Autodesk Inventor part; units mm, degrees
ref_plane "YZ Plane" through (0, 0, 0) normal (1, 0, 0) x (0, 1, 0)
ref_plane "XZ Plane" through (0, 0, 0) normal (0, 1, 0) x (-1, 0, 0)
ref_plane "XY Plane" through (0, 0, 0) normal (0, 0, 1) x (1, 0, 0)
sketch "Sketch1" plane through (0, 0, 0) normal (0, 0, 1) x (1, 0, 0)
  line L0 (25.4, -76.2) -> (25.4, 76.2)
  line L1 (25.4, 76.2) -> (-25.4, 76.2)
  line L2 (-25.4, 76.2) -> (-25.4, -76.2)
  line L3 (-25.4, -76.2) -> (25.4, 76.2) construction
  line L4 (25.4, -76.2) -> (-25.4, 76.2) construction
  line L5 (29.3687, -76.2) -> (29.3687, 80.1688)
  line L6 (29.3687, 80.1688) -> (-29.3687, 80.1688)
  line L7 (-29.3687, 80.1688) -> (-29.3687, -76.2)
  line L8 (-29.3687, -80.1688) -> (29.3687, 80.1688) construction
  line L9 (29.3687, -80.1688) -> (-29.3687, 80.1688) construction
  line L10 (-25.4, -76.2) -> (-29.3687, -76.2)
  line L11 (25.4, -76.2) -> (29.3687, -76.2)
  point P0 (0, 0)
  dimension "d2" = 3.9688
  dimension "d3" = 3.9688
  dimension "d5" = 50.8
  dimension "d6" = 152.4
extrude "Extrusion1" add sketch "Sketch1" along normal blind 31.75
sketch "Sketch2" plane through (0, 0, 0) normal (0, 0, -1) x (-1, 0, 0)
  line L0 (-29.3687, -76.2) -> (-29.3687, 80.1688)
  line L1 (29.3687, 80.1688) -> (29.3687, -76.2)
  line L2 (-29.3687, 80.1688) -> (29.3687, 80.1688)
  line L3 (29.3687, 80.1688) -> (29.3687, -76.2)
  line L4 (29.3687, -76.2) -> (-29.3687, -76.2)
  line L5 (-29.3687, -76.2) -> (-29.3687, 80.1688)
  point P0 (0, 0)
extrude "Extrusion2" add sketch "Sketch2" along normal blind 3.9688
sketch "Sketch5" plane through (0, 0, 31.75) normal (0, 0, 1) x (1, 0, 0)
  line L0 (-29.3687, 80.1688) -> (-29.3687, -76.2)
  line L1 (-29.3687, 42.0688) -> (-46.7574, 42.0688) construction
  line L2 (-29.3687, 31.9088) -> (-46.7574, 31.9088)
  line L3 (-46.7574, 52.2287) -> (-29.3687, 52.2288)
  arc A0 (-46.7574, 52.2287) -> (-46.7574, 31.9088) centre (-46.7574, 42.0688) ccw
  line L4 (29.3687, 80.1688) -> (-29.3687, 80.1688)
  circle A1 centre (-46.7574, 42.0688) radius 2.54
  point P0 (0, 0)
  dimension "d18" = 10.16
  dimension "d21" = 5.08
extrude "Extrusion4" add sketch "Sketch5" against normal blind 3.9688
mirror "Mirror1" about plane through (0, 0, 0) normal (1, 0, 0) of "Extrusion4"
mirror "Mirror2" about plane through (0, 0, 0) normal (0, 1, 0) of "Extrusion4", "Mirror1"
sketch "Sketch6" plane through (0, 0, 0) normal (0, 0, 1) x (1, 0, 0)
  circle A0 centre (-12.7, -63.5) radius 1.5875
  line L0 (-25.4, -76.2) -> (-25.4, 76.2)
  line L1 (-25.4, -76.2) -> (25.4, -76.2) construction
  line L2 (-12.7, -63.5) -> (-12.7, 76.2) construction
  line L3 (-25.4, 76.2) -> (25.4, 76.2) construction
  line L4 (-12.7, -63.5) -> (25.4, -63.5) construction
  circle A1 centre (-12.7, -50.8) radius 1.5875
  circle A2 centre (-12.7, -38.1) radius 1.5875
  circle A3 centre (-12.7, -25.4) radius 1.5875
  circle A4 centre (-12.7, -12.7) radius 1.5875
  circle A5 centre (-12.7, 0) radius 1.5875
  circle A6 centre (-12.7, 12.7) radius 1.5875
  circle A7 centre (-12.7, 25.4) radius 1.5875
  circle A8 centre (-12.7, 38.1) radius 1.5875
  circle A9 centre (-12.7, 50.8) radius 1.5875
  circle A10 centre (-12.7, 63.5) radius 1.5875
  circle A11 centre (0, -63.5) radius 1.5875
  circle A12 centre (0, -50.8) radius 1.5875
  circle A13 centre (0, -38.1) radius 1.5875
  circle A14 centre (0, -25.4) radius 1.5875
  circle A15 centre (0, -12.7) radius 1.5875
  circle A16 centre (0, 0) radius 1.5875
  circle A17 centre (0, 12.7) radius 1.5875
  circle A18 centre (0, 25.4) radius 1.5875
  circle A19 centre (0, 38.1) radius 1.5875
  circle A20 centre (0, 50.8) radius 1.5875
  circle A21 centre (0, 63.5) radius 1.5875
  circle A22 centre (12.7, -63.5) radius 1.5875
  circle A23 centre (12.7, -50.8) radius 1.5875
  circle A24 centre (12.7, -38.1) radius 1.5875
  circle A25 centre (12.7, -25.4) radius 1.5875
  circle A26 centre (12.7, -12.7) radius 1.5875
  circle A27 centre (12.7, 0) radius 1.5875
  circle A28 centre (12.7, 12.7) radius 1.5875
  circle A29 centre (12.7, 25.4) radius 1.5875
  circle A30 centre (12.7, 38.1) radius 1.5875
  circle A31 centre (12.7, 50.8) radius 1.5875
  circle A32 centre (12.7, 63.5) radius 1.5875
  dimension "d24" = 3.175
  dimension "d25" = 12.7
  dimension "d26" = 12.7
  dimension "d29" = 12.7
  dimension "d32" = 12.7
extrude "Extrusion5" cut sketch "Sketch6" against normal through all
equation "\"d2\" = wallThickness"
equation "\"d3\" = wallThickness"
equation "\"d5\" = interiorWidth"
equation "\"d6\" = interiorHeight"
equation "\"d7\" = interiorDepth"
equation "\"d9\" = wallThickness"
equation "\"d18\" = tabWidth"
equation "\"d21\" = screwHole"
equation "\"d22\" = wallThickness"
equation "\"interiorWidth\" = 50.8"
equation "\"interiorHeight\" = 152.4"
equation "\"wallThickness\" = 3.96875"
equation "\"interiorDepth\" = 31.75"
equation "\"screwHole\" = 5.08"
equation "\"tabWidth\" = 10.16"
properties part number "thermometerCover"
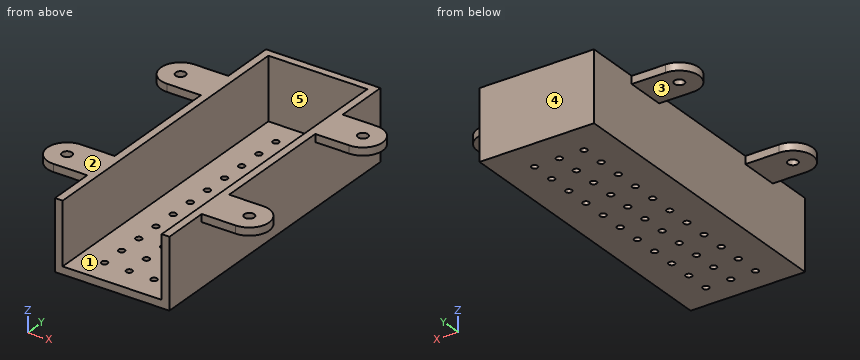
Source: CAD feature listing. Evaluate the final solid. Frame: model axes, mm. Face numbers are marked on the shaded views. A direction names the side the tool comes from. Give positions to 0.01 mm unless a question says otherwise; leave off trailing zeros. Loops run counter-clockwise (first coordinate to the right, second up) from the corner with the lowest first, then second, coordinate; pieces in that order, holes last. Notation, with made-up numbers: (85.5, -16.75) -> (133.5, -16.75) arc R25 ccw to (133.5, 17.25) -> close; hole circle Ø4 at (45.5, 54.25). An arc over 180 degrees is marked (long way). Put each result on its own line as item: value. Start each with the question number.
1) Draft query along X for the marked faces 1 and 2. Return one class per face: released by +X, released by -X, zero draft, split by the parting line, or undercut.
2) Cut plane C-C (z = 29.5). Return loops of the section in (x, y).
3) Cut plane A-A (y = 63.5). Return loops of the section in (x, z).
4) Material intervals for probe 1 along X at (y, z) = (-15, 6); probe 2 along X at (y, z) = (38, -2); probe 3 along Y at (x, z) = (-25, 20), sorted ascending.
5) Contact query for flat-ended pins moving along their axis: P1, Ø1.9, axis at x = 0, y = 50.8, coming from the -Z side; P2, Ø3, axis at x = -42, z = 30.5, coming from the +Y side; P3, Ø12, axis at x = 8, z = 24.5, coming from the -Y side; P4, Ø8, axis at y = 63.5, z = 3.5, coming from the +X side. Output: stop coordinate, or through.
6) Reachability of the marked faces 3, 4 and 5 from +Z, -Z, +X, -X, +Y, -Y: full face, straight path, thin tool, end or side. Return the list, or none.
7) Cut plane B-B (x = 41). Return loops of the section in (y, z), then the cut area to 3 significant figures.
8) Cut plane D-D (x = -7.5). Return loops of the section in (y, z).
Results are:
1. face 1: undercut
1. face 2: zero draft
2. outline: (-46.76, -52.23) -> (-29.37, -52.23) -> (-29.37, -76.2) -> (-25.4, -76.2) -> (-25.4, 76.2) -> (25.4, 76.2) -> (25.4, -76.2) -> (29.37, -76.2) -> (29.37, -52.23) -> (46.76, -52.23) arc R10.16 ccw to (46.76, -31.91) -> (29.37, -31.91) -> (29.37, 31.91) -> (46.76, 31.91) arc R10.16 ccw to (46.76, 52.23) -> (29.37, 52.23) -> (29.37, 80.17) -> (-29.37, 80.17) -> (-29.37, 52.23) -> (-46.76, 52.23) arc R10.16 ccw to (-46.76, 31.91) -> (-29.37, 31.91) -> (-29.37, -31.91) -> (-46.76, -31.91) arc R10.16 ccw to start; hole circle Ø5.08 at (-46.76, -42.07); hole circle Ø5.08 at (-46.76, 42.07); hole circle Ø5.08 at (46.76, -42.07); hole circle Ø5.08 at (46.76, 42.07)
3. outline: (-29.37, -3.97) -> (-14.29, -3.97) -> (-14.29, 0) -> (-25.4, 0) -> (-25.4, 31.75) -> (-29.37, 31.75) -> close; (-11.11, -3.97) -> (-1.59, -3.97) -> (-1.59, 0) -> (-11.11, 0) -> close; (1.59, -3.97) -> (11.11, -3.97) -> (11.11, 0) -> (1.59, 0) -> close; (14.29, -3.97) -> (29.37, -3.97) -> (29.37, 31.75) -> (25.4, 31.75) -> (25.4, 0) -> (14.29, 0) -> close
4. probe 1: x = -29.37 to -25.4, 25.4 to 29.37
4. probe 2: x = -29.37 to -14.28, -11.12 to -1.58, 1.58 to 11.12, 14.28 to 29.37
4. probe 3: y = 76.2 to 80.17
5. P1: passes through
5. P2: stops at y = 52.23
5. P3: stops at y = 76.2
5. P4: stops at x = 29.37
6. face 3: -Z, -X, +Y, -Y
6. face 4: +Z, -Z, +X, -X, +Y
6. face 5: +Z, -Y
7. outline: (-52.23, 27.78) -> (-31.91, 27.78) -> (-31.91, 31.75) -> (-52.23, 31.75) -> close; (31.91, 27.78) -> (52.23, 27.78) -> (52.23, 31.75) -> (31.91, 31.75) -> close
7. area: 161 mm2
8. outline: (-76.2, -3.97) -> (80.17, -3.97) -> (80.17, 31.75) -> (76.2, 31.75) -> (76.2, 0) -> (-76.2, 0) -> close
